Here's the drawing with two shaded views (mm, measured from the low corner). I have some questions. Round coordinates to 2 decimals unless told otherwise and drop trailing zeros. Order: outer loops, then holes, each group sorted by start corner. A loop starts at its lowest first (then second) coordinate and runs counter-clockwise, first axis right, second up.
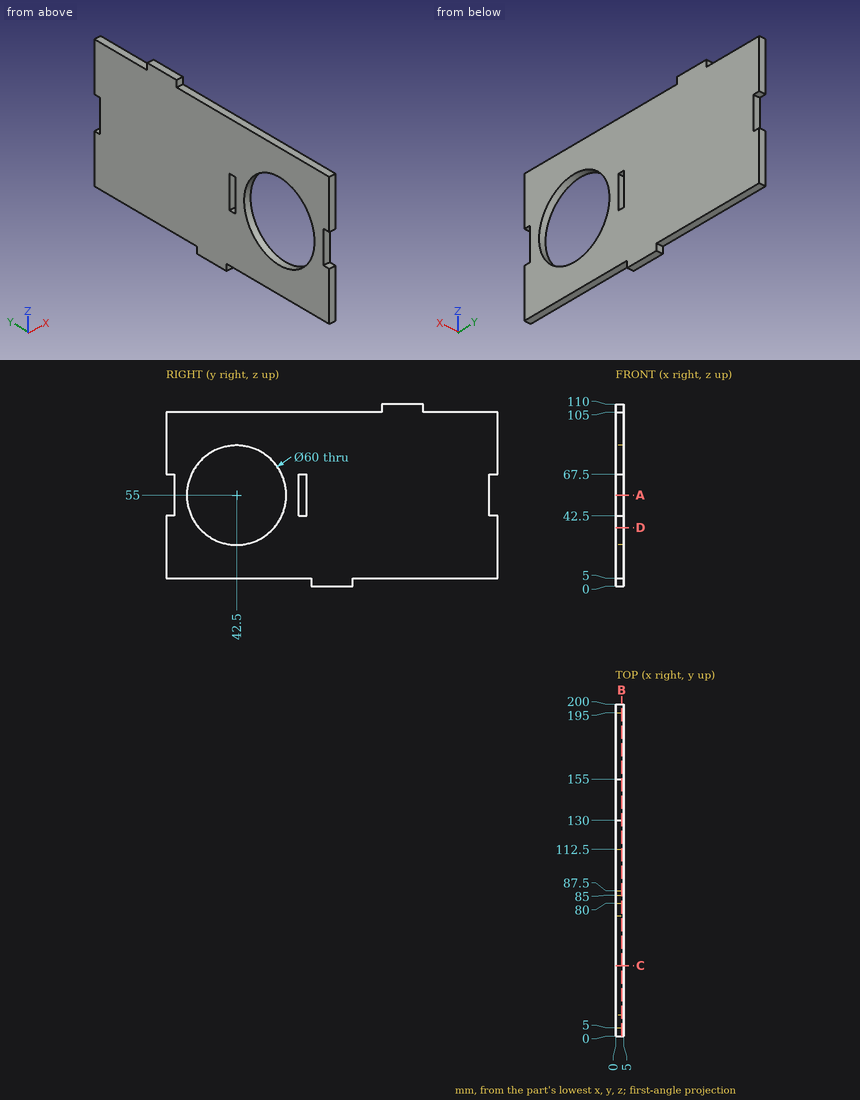
1. If we section it at A-A, the plane z = 55: Write out the boundary of the cut face in (x, y), and give its area (3 significant figures).
Evaluation:
outline: (0, 5) - (5, 5) - (5, 12.5) - (0, 12.5) - close; (0, 72.5) - (5, 72.5) - (5, 80) - (0, 80) - close; (0, 85) - (5, 85) - (5, 195) - (0, 195) - close
area: 625 mm2
2. If we section it at D-D, the plane z = 35.5: Write out the boundary of the cut face in (x, y), and give its area (3 significant figures).
Evaluation:
outline: (0, 0) - (5, 0) - (5, 19.7) - (0, 19.7) - close; (0, 65.3) - (5, 65.3) - (5, 200) - (0, 200) - close
area: 772 mm2
3. If we section it at C-C, the plane y = 42.5: Write out the boundary of the cut face in (x, z), and give its area (3 significant figures).
Evaluation:
outline: (0, 5) - (5, 5) - (5, 25) - (0, 25) - close; (0, 85) - (5, 85) - (5, 105) - (0, 105) - close
area: 200 mm2
4. If we section it at B-B, the plane x = 3.6: Write out the boundary of the cut face in (y, z), and give its area (3 significant figures).
Evaluation:
outline: (0, 5) - (87.5, 5) - (87.5, 0) - (112.5, 0) - (112.5, 5) - (200, 5) - (200, 42.5) - (195, 42.5) - (195, 67.5) - (200, 67.5) - (200, 105) - (155, 105) - (155, 110) - (130, 110) - (130, 105) - (0, 105) - (0, 67.5) - (5, 67.5) - (5, 42.5) - (0, 42.5) - close; hole circle Ø60 at (42.5, 55); hole (80, 42.5) - (85, 42.5) - (85, 67.5) - (80, 67.5) - close
area: 17,000 mm2
5. I need wall thicknesses on probe 1 along Z at (x, y) = (1.6, 42.5); probe 2 along Y at (x, z) = (0.7, 64.5); probe 3 along Z at (x, y) = (2, 17). Which ranges of each line are inside material? Lowest first, please.
Evaluation:
probe 1: z = 5 to 25, 85 to 105
probe 2: y = 5 to 14.04, 70.96 to 80, 85 to 195
probe 3: z = 5 to 39.2, 70.8 to 105
6. I'm going to push flat-ended pins straight in: P1, Ø1.5, axis at x = 2, y = 46, coming from the +Z side; P2, Ø1.5, axis at x = 2.5, z = 3, coming from the -Y side; P3, Ø2.5, axis at x = 1.5, y = 82.5, coming from the -Z side. Where does each tip first touch, or does it pass through?
Evaluation:
P1: stops at z = 105
P2: stops at y = 87.5
P3: stops at z = 5
